from build123d import *

# Parameters (mm, degrees)
SKETCH002_R        = 12.2
PAD_DEPTH          = 3
POCKET_DEPTH       = 3.001
SKETCH003_W        = 1.3
SKETCH003_H        = 3
POCKET001_DEPTH    = 72.274949
POLARPATTERN_COUNT = 20
CHAMFER_SIZE       = 0.5


with BuildPart() as part:
    # Sketch002 → Pad (new body)
    with BuildSketch(Plane.XY):
        Circle(SKETCH002_R)
    extrude(amount=PAD_DEPTH)

    # Sketch → Pocket (cut, through all)
    with BuildSketch(Plane.XY.offset(3)):
        with BuildLine():
            Line((-2.12132, 1.75), (2.12132, 1.75))
            ThreePointArc((2.12132, -1.75), (2.75, 0), (2.12132, 1.75))
            Line((-2.12132, -1.75), (2.12132, -1.75))
            ThreePointArc((-2.12132, 1.75), (-2.75, 0), (-2.12132, -1.75))
        make_face()
    extrude(amount=-POCKET_DEPTH, mode=Mode.SUBTRACT)

    # Sketch003 → Pocket001 (cut, through all)
    with BuildSketch(Plane.XY.offset(3)):
        with Locations((0, 8.7)):
            Rectangle(SKETCH003_W, SKETCH003_H)
    pocket001 = extrude(amount=-POCKET001_DEPTH, mode=Mode.SUBTRACT)

    # PolarPattern: Pocket001 ×20 about axis
    polarpattern_axis = Axis((0, 0, 3), (0, 0, 1))
    for i in range(1, POLARPATTERN_COUNT):
        add(pocket001.rotate(polarpattern_axis, i * 360 / POLARPATTERN_COUNT), mode=Mode.SUBTRACT)

    # Chamfer
    chamfer_edges = [part.edges().sort_by_distance(p)[0] for p in [
        (-2.75, 0, 3),
        (0, 1.75, 3),
        (2.75, 0, 3),
        (0, -1.75, 3),
        (-12.2, 0, 3),
        (-12.2, 0, 0),
        (-2.75, 0, 0),
        (0, 1.75, 0),
        (0, -1.75, 0),
        (2.75, 0, 0),
    ]]
    chamfer(chamfer_edges, length=CHAMFER_SIZE)


solid = part.part
Here's how the part is built. I have some questions about the finished solid (model axes, mm). A direction names the side the tool comes from. Give positions to 0.01 mm unless a question says otherwise; leave off trailing zeros. Order: outer loops, then holes, each group sorted by start corner. A loop starts at its lowest first (then second) coordinate and runs counter-clockwise, first axis right, second up. Notation, with made-up numbers: (60.25, -8) -> (105.25, -8) arc R10 cw to (105.25, -2) -> close; hole circle Ø6 at (-12.5, 8). An arc over 180 degrees is marked (long way). One line per item, written item: value. Start each with the question number.
1. Will these pins go through, and if not, where does the flat tip stop? pin 1 Ø0.9 at (y, z) = (8.5, 1.5) entering from -X; pin 2 Ø0.9 at (x, z) = (-9.5, 1.5) entering from -Y; pin 3 Ø1.5 at (y, z) = (-2.5, 0.5) entering from +X.
2. I need wall thicknesses on probe 1 along X at (y, z) = (-0.5, 2.6); probe 2 along X at (y, z) = (9, 1); probe 3 along X at (y, z) = (4.5, 2.55). Which ranges of each line are inside material? Lowest first, please. Write a range as from..to.
3. We'd pull the mould along Y, two halves only. Please class faces 3 (the face through (0, -10.2, 2)), 4 (the face through (-12.19, 0.54, 1.49)), 5 (the face through (-6.6, -5.6, 1.5)): released by +Y, released by -Y, zero draft, split by the parting line, or undercut.
4. Imagine slicing it at A-A, the plane x = 0. List the corners of the cut face in (y, z) for me, plus the area to 3 significant figures.
5. Imagine slicing it at C-C, the plane z = 2.15. Count the separate pieces of the cut face and the enclosed holes in it, plus the area to 3 significant figures.
6. Imagine slicing it at B-B, the plane y = 0. List the corners of the cut face in (x, z) for me.
7. For faces 1 (the face through (-8.05, 3.3, 1.52)), 2 (the face through (-2.89, 0.03, 2.64)), which set-ups out of +Z, -Z, +X, -X, +Y, -Y let a thin tool reach every point of the face, with its end or its side?
Values follow:
1. pin 1: stops at x = -9.17
1. pin 2: stops at y = -8.18
1. pin 3: stops at x = 12.07
2. probe 1: x = -12.09..-10.2, -7.2..-2.81, 2.81..7.2, 10.2..12.09
2. probe 2: x = -8.24..-3.61, -2.24..-0.65, 0.65..2.24, 3.61..8.24
2. probe 3: x = -11.29..-7.3, -5.63..5.63, 7.3..11.29
3. face 3: undercut
3. face 4: split by the parting line
3. face 5: undercut
4. outline: (-12.2, 0.5) -> (-11.7, 0) -> (-10.2, 0) -> (-10.2, 3) -> (-11.7, 3) -> (-12.2, 2.5) -> close; (-7.2, 0) -> (-2.25, 0) -> (-1.75, 0.5) -> (-1.75, 2.5) -> (-2.25, 3) -> (-7.2, 3) -> close; (1.75, 0.5) -> (2.25, 0) -> (7.2, 0) -> (7.2, 3) -> (2.25, 3) -> (1.75, 2.5) -> close; (10.2, 0) -> (11.7, 0) -> (12.2, 0.5) -> (12.2, 2.5) -> (11.7, 3) -> (10.2, 3) -> close
4. area: 43.7 mm2
5. separate pieces: 1
5. enclosed holes: 21
5. area: 372 mm2
6. outline: (-12.2, 0.5) -> (-11.7, 0) -> (-10.2, 0) -> (-10.2, 3) -> (-11.7, 3) -> (-12.2, 2.5) -> close; (-7.2, 0) -> (-3.25, 0) -> (-2.75, 0.5) -> (-2.75, 2.5) -> (-3.25, 3) -> (-7.2, 3) -> close; (2.75, 0.5) -> (3.25, 0) -> (7.2, 0) -> (7.2, 3) -> (3.25, 3) -> (2.75, 2.5) -> close; (10.2, 0) -> (11.7, 0) -> (12.2, 0.5) -> (12.2, 2.5) -> (11.7, 3) -> (10.2, 3) -> close
7. face 1: +Z, -Z
7. face 2: +Z
